```python
from build123d import *

# Parameters (mm, degrees)
SKETCH_1_R          = 34
EXTRUDE_1_DEPTH     = 22
SKETCH_2_R          = 26
CUT_EXTRUDE_1_DEPTH = 22
FILLET_1_R          = 4


with BuildPart() as part:
    # 草图1 → 凸台-拉伸1 (new body)
    with BuildSketch(Plane(origin=(0, 0, 0), x_dir=(0, 0, -1), z_dir=(1, 0, 0))):
        Circle(SKETCH_1_R)
    extrude(amount=EXTRUDE_1_DEPTH)

    # 草图2 → 切除-拉伸1 (cut)
    with BuildSketch(Plane.ZY):
        Circle(SKETCH_2_R)
    extrude(amount=-CUT_EXTRUDE_1_DEPTH, mode=Mode.SUBTRACT)

    # 圆角1
    fillet_1_edges = [part.edges().sort_by_distance(p)[0] for p in [
        (0, 0, 34),
        (22, 0, 34),
    ]]
    fillet(fillet_1_edges, radius=FILLET_1_R)


solid = part.part
```
Input: part model. Units: mm. Frame: model coordinates. Round coordinates to 2 decimals unless told otherwise and drop trailing zeros. Loops run counter-clockwise (first coordinate to the right, second up) from the corner with the lowest first, then second, coordinate; pieces in that order, holes last. Notation, with made-up numbers: M -37,27.25 L 20,27.25 A18 cw 20,33.25 Z; hole C -28.75,34 d10. An arc over 180 degrees is marked long. Answer in a Markdown table with one row per item. Add a question column.
1. Mould query, pull axis Z, two halves, no side actions, for faces 1 (the face through (10.9, 28.67, -18.28)), 2 (the face through (10.846, -15.821, -20.633)), 3 (the face through (22, 25, 9)). Classes: released by +Z, released by -Z, zero draft, split by the parting line, or undercut.
2. Contact query for flat-ended pins moving along their axis: pin 1 (12 mm diameter, centred on x = 2.5, z = -20, fed in from -Y); pin 2 (4 mm diameter, centred on x = 17, z = 16.5, fed in from -Y); pin 3 (6 mm diameter, centred on x = 12.5, z = 18.5, fed in from +Y). Output: stop coordinate, or through.
3. Section A-A (y = 0). Output: boundary loops of the cut face in (x, z).
4. Section C-C (x = 16.5). Output: boundary loops of the cut face in (y, z), and give its area (3 significant figures).
5. Ray query, probe 1 along Y at (x, z) = (13, 0); probe 2 along Y at (x, z) = (3.25, -2); probe 3 along Z at (x, y) = (5.5, -2.5). Return the intervals inside material, ascending.
6. Section D-D (x = 1.5). Output: boundary loops of the cut face in (y, z) (1 decimal), and give its area (3 significant figures).
Values follow:
| question | item | result |
|---|---|---|
| 1 | face 1 | split by the parting line |
| 1 | face 2 | undercut |
| 1 | face 3 | zero draft |
| 2 | pin 1 | y = -30.92 |
| 2 | pin 2 | y = -30.75 |
| 2 | pin 3 | y = 30.26 |
| 3 | outline | M 0,-30 A4 ccw 4,-34 L 18,-34 A4 ccw 22,-30 L 22,-26 L 0,-26 Z; M 0,26 L 22,26 L 22,30 A4 ccw 18,34 L 4,34 A4 ccw 0,30 Z |
| 4 | outline | C 0,0 d68; hole C 0,0 d52 |
| 4 | area | 1,510 mm^2 |
| 5 | probe 1 | -34 to -26, 26 to 34 |
| 5 | probe 2 | -33.87 to -25.92, 25.92 to 33.87 |
| 5 | probe 3 | -33.91 to -25.88, 25.88 to 33.91 |
| 6 | outline | C 0,0 d66.2; hole C 0,0 d52 |
| 6 | area | 1,320 mm^2 |
